The listing builds one solid part. Answer for the finished solid, in the listing's coordinates (mm). Face numbers are marked on the shaded views. A direction names the side the tool comes from. Coordinates: 2 decimals unless noted, no trailing zeros. Write each loop counter-clockwise with the first axis right and the second up, starting at its lowest first coordinate (ties: lowest second). Pieces come first, ordered by that corner, then holes.
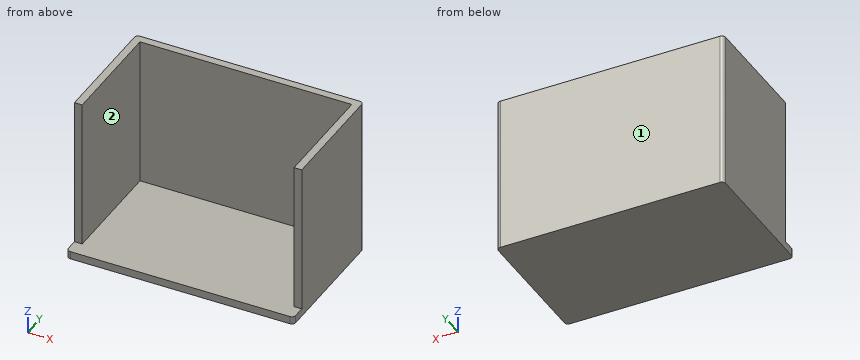
from build123d import *

# Parameters (mm, degrees)
F1_DEPTH = 19.05
F0_W     = 19.05
F0_H     = 273.05
F2_DEPTH = 387.35
F3_R     = 9.525


with BuildPart() as f1:
    # F0 (on Top) → F1 (new body)
    with BuildSketch(Plane.XY):
        Polygon((0, 38.1), (0, 0), (558.8, 0), (558.8, 38.1), (539.75, 38.1), (539.75, 311.15), (19.05, 311.15), (19.05, 38.1), align=None)
    extrude(amount=F1_DEPTH)

    # F0 (on Top) → F2 (join)
    with BuildSketch(Plane.XY):
        Polygon((0, 330.2), (0, 311.15), (19.05, 311.15), (539.75, 311.15), (558.8, 311.15), (558.8, 330.2), align=None)
        with Locations((9.525, 174.625)):
            Rectangle(F0_W, F0_H)
        with Locations((549.275, 174.625)):
            Rectangle(F0_W, F0_H)
    extrude(amount=F2_DEPTH)

    # F3
    f3_edges = [f1.edges().sort_by_distance(p)[0] for p in [
        (0, 330.2, 193.675),
        (558.8, 330.2, 193.675),
        (558.8, 0, 9.525),
        (0, 0, 9.525),
    ]]
    fillet(f3_edges, radius=F3_R)


solid = f1.part
1. Section A-A on y = 51.5 is taken. Give the vertices of the cut face in (x, z).
Results found:
outline: (0, 0) - (558.8, 0) - (558.8, 387.35) - (539.75, 387.35) - (539.75, 19.05) - (19.05, 19.05) - (19.05, 387.35) - (0, 387.35) - close
2. A tool of negligible diameter and unlimited length cuts with its end or side. For the marked faces 1 and 2, from which of +Z, -Z, +X, -X, +Y, -Y can it reach the whole face along a straight path? Write none if from no direction.
Results found:
face 1: +Z, -Z, +X, -X, +Y
face 2: +Z, -Y
3. Section B-B on z = 141 is taken. Give the vertices of the cut face in (x, y) (3 decimals), then the cut area to 3 significant figures.
Results found:
outline: (0, 38.1) - (19.05, 38.1) - (19.05, 311.15) - (539.75, 311.15) - (539.75, 38.1) - (558.8, 38.1) - (558.8, 320.675) arc R9.525 ccw to (549.275, 330.2) - (9.525, 330.2) arc R9.525 ccw to (0, 320.675) - close
area: 21,000 mm2
4. Find the intervals of material crossed by L1, parallel to X at y = 208, z = 229; L2, parallel to Z at x = 67, y = 179; L3, parallel to Y at x = 129.5, z = 215, in increasing order.
Results found:
L1: x = 0 to 19.05, 539.75 to 558.8
L2: z = 0 to 19.05
L3: y = 311.15 to 330.2
5. Section C-C on x = 378 is taken. Give the vertices of the cut face in (y, z), then the cut area to 3 significant figures.
Results found:
outline: (0, 0) - (330.2, 0) - (330.2, 387.35) - (311.15, 387.35) - (311.15, 19.05) - (0, 19.05) - close
area: 13,300 mm2
6. Flat-ended cylindrical pins translate along their axes: P1, Ø1.5, axis at x = 64.5, y = 80.5, coming from the +Z side; P2, Ø6, axis at x = 345, z = 81.5, coming from the -Y side; P3, Ø5.5, axis at x = 9, z = 235.5, coming from the -Y side. Find the tip coordinate at first contact, or state that the pin passes through.
Results found:
P1: stops at z = 19.05
P2: stops at y = 311.15
P3: stops at y = 38.1
